from build123d import *

# Parameters (mm, degrees)
SKIZZE1_R                              = 14.5
AUFSATZ_LINEAR_AUSTRAGEN1_DEPTH        = 50
SKIZZE5_W                              = 3.2
SKIZZE5_H                              = 2
SCHNITT_LINEAR_AUSTRAGEN1_DEPTH        = 25
F_24_5_24_5_DURCHMESSER_BOHRUNG1_D     = 12.5
F_24_5_24_5_DURCHMESSER_BOHRUNG2_D     = 25
F_24_5_24_5_DURCHMESSER_BOHRUNG2_DEPTH = 30
F_24_5_24_5_DURCHMESSER_BOHRUNG2_TIP   = 7.510757738
SCHNITT_LINEAR_AUSTRAGEN2_DEPTH        = 20
F_2_0_2_DURCHMESSER_BOHRUNG11_D        = 2
F_2_0_2_DURCHMESSER_BOHRUNG11_DEPTH    = 30
F_2_0_2_DURCHMESSER_BOHRUNG11_TIP      = 0.600860619


with BuildPart() as part:
    # Skizze1 → Aufsatz-Linear austragen1 (new body)
    with BuildSketch(Plane.XY):
        Circle(SKIZZE1_R)
    extrude(amount=AUFSATZ_LINEAR_AUSTRAGEN1_DEPTH)

    # Skizze5 → Schnitt-Linear austragen1 (cut)
    with BuildSketch(Plane(origin=(0, 0, 0), x_dir=(-1, 0, 0), z_dir=(0, 0, -1))):
        with Locations((0, 6.8)):
            Rectangle(SKIZZE5_W, SKIZZE5_H)
    extrude(amount=-SCHNITT_LINEAR_AUSTRAGEN1_DEPTH, mode=Mode.SUBTRACT)

    # Ø24.5 (24.5) Durchmesser Bohrung1 (through all)
    with Locations(Plane(origin=(0, 0, 0), x_dir=(-1, 0, 0), z_dir=(0, 0, -1))):
        with Locations((0, 0)):
            Hole(F_24_5_24_5_DURCHMESSER_BOHRUNG1_D / 2)

    # Ø24.5 (24.5) Durchmesser Bohrung2
    with Locations(Plane.XY.offset(50)):
        with Locations((0, 0)):
            Hole(F_24_5_24_5_DURCHMESSER_BOHRUNG2_D / 2, depth=F_24_5_24_5_DURCHMESSER_BOHRUNG2_DEPTH)
            with Locations((0, 0, -(F_24_5_24_5_DURCHMESSER_BOHRUNG2_DEPTH + F_24_5_24_5_DURCHMESSER_BOHRUNG2_TIP / 2))):  # 118° drill point
                Cone(0, F_24_5_24_5_DURCHMESSER_BOHRUNG2_D / 2, F_24_5_24_5_DURCHMESSER_BOHRUNG2_TIP, mode=Mode.SUBTRACT)

    # Skizze12 → Schnitt-Linear austragen2 (cut)
    with BuildSketch(Plane.XY.offset(50)):
        with BuildLine():
            Line((-14.491376746, 0.5), (-12.489995997, 0.5))
            ThreePointArc((-12.489995997, 0.5), (-12.5, 0), (-12.489995997, -0.5))
            Line((-12.489995997, -0.5), (-14.491376746, -0.5))
            ThreePointArc((-14.491376746, -0.5), (-14.5, 0), (-14.491376746, 0.5))
        make_face()
        with BuildLine():
            Line((12.489995997, 0.5), (14.491376746, 0.5))
            ThreePointArc((14.491376746, 0.5), (14.5, 0), (14.491376746, -0.5))
            Line((14.491376746, -0.5), (12.489995997, -0.5))
            ThreePointArc((12.489995997, -0.5), (12.5, 0), (12.489995997, 0.5))
        make_face()
    extrude(amount=-SCHNITT_LINEAR_AUSTRAGEN2_DEPTH, mode=Mode.SUBTRACT)

    # Ø2.0 (2) Durchmesser Bohrung11
    with Locations(Plane(origin=(-14.5, 0, 30), x_dir=(0, 0, 1), z_dir=(-1, 0, 0))):
        with Locations((0, 0)):
            Hole(F_2_0_2_DURCHMESSER_BOHRUNG11_D / 2, depth=F_2_0_2_DURCHMESSER_BOHRUNG11_DEPTH)
            with Locations((0, 0, -(F_2_0_2_DURCHMESSER_BOHRUNG11_DEPTH + F_2_0_2_DURCHMESSER_BOHRUNG11_TIP / 2))):  # 118° drill point
                Cone(0, F_2_0_2_DURCHMESSER_BOHRUNG11_D / 2, F_2_0_2_DURCHMESSER_BOHRUNG11_TIP, mode=Mode.SUBTRACT)


solid = part.part
The listing builds one solid part. Answer for the finished solid, in the listing's coordinates (mm). A direction names the side the tool comes from. Round coordinates to 2 decimals unless told otherwise and drop trailing zeros. Write each loop counter-clockwise with the first axis right and the second up, starting at its lowest first coordinate (ties: lowest second). Pieces come first, ordered by that corner, then holes. Notation, with made-up numbers: (-16, 41.5) - (11, 41.5) arc R12 ccw to (11, 57.5) - close; hole circle Ø4 at (2.5, 50.25). An arc over 180 degrees is marked (long way). Use one line per item in the form item = value. Start each with the question number.
Item 1: Find the intervals of material crossed by line 1 (Y direction, x = 0, z = 30); line 2 (X direction, y = 0, z = 9.25); line 3 (Y direction, x = 0, z = 8.5), in increasing order. Write a range as [from, to].
Item 2: A cutting plane is placed at A-A (z = 31.5). Write down the section's boundary in (x, y).
Item 3: Determine the mould class of faces 4 (the cylindrical face through (13.83, 4.36, 24.65)), 5 (the flat face through (0, 7.8, 9)), 6 (the flat face through (3, -6, 0)) for opening direction X: +X half, -X half, draft (parallel to the pull), parting line (faces both ways), or undercut.
Item 4: A tool of negligible diameter and unlimited length cuts with its end or side. For faces 1 (the flat face through (-14, 0.5, 41)), 2 (the cylindrical face through (-11.923, 3.755, 34.79)), 3 (the flat face through (1.6, 7, 9)), from which of +Z, -Z, +X, -X, +Y, -Y can it reach the whole face along a straight path? Write none if from no direction.
Item 5: Flat-ended cylindrical pins translate along their axes: pin 1 Ø1.6 at (x, z) = (-13.5, 41) entering from +Y; pin 2 Ø4 at (x, y) = (0.5, 11) entering from -Z; pin 3 Ø2 at (x, y) = (3.5, -0.5) entering from -Z; pin 4 Ø10 at (x, z) = (-9.5, 36) entering from +Y. Find the tip coordinate at first contact, or state that the pin passes through.
Item 6: A cutting plane is placed at B-B (x = 0). Write down the section's boundary in (y, z), plus the area to 3 significant figures.
Item 7: A cutting plane is placed at C-C (z = 10.5). Write down the section's boundary in (x, y).
The answers:
q1.line_1 = [-14.5, -12.5], [12.5, 14.5]
q1.line_2 = [-14.5, -6.25], [6.25, 14.5]
q1.line_3 = [-14.5, -6.25], [7.8, 14.5]
q2.outline = (-14.49, -0.5) arc R14.5 ccw to (14.49, -0.5) - (12.49, -0.5) arc R12.5 cw to (-12.49, -0.5) - close; (-14.49, 0.5) - (-12.49, 0.5) arc R12.5 cw to (12.49, 0.5) - (14.49, 0.5) arc R14.5 ccw to start
q3.face_4 = parting line
q3.face_5 = undercut
q3.face_6 = draft
q4.face_1 = +Z, +X, -X
q4.face_2 = +Z
q4.face_3 = +Z, -Z
q5.pin_1 = 7
q5.pin_2 = 0
q5.pin_3 = through
q5.pin_4 = 13.78
q6.outline = (-14.5, 0) - (-6.25, 0) - (-6.25, 16.24) - (-12.5, 20) - (-12.5, 50) - (-14.5, 50) - close; (7.8, 0) - (14.5, 0) - (14.5, 50) - (12.5, 50) - (12.5, 20) - (7.8, 17.18) - close
q6.area = 401 mm^2
q7.outline = circle Ø29 at (0, 0); hole (-1.6, 6.04) arc R6.25 ccw (long way) to (1.6, 6.04) - (1.6, 7.8) - (-1.6, 7.8) - close
